Study the drawing (mm; zero at the part's minimum x, y, z) and answer. Coordinates: 2 decimals unless noted, no trailing zeros. Order: outer loops, then holes, each group sorted by start corner. A loop starts at its lowest first (then second) coordinate and runs counter-clockwise, first axis right, second up. Notation, with made-up numbers: M 62.5,73.5 L 67.5,73.5 A14 ccw 67.5,81.5 Z; hole C 86.5,5.25 d10. An arc over 180 degrees is marked long. One line per item, written item: value. Start each with the question number.
Q1. Straight lines are drawn through the part: line 1 along Z through (x, y) = (7, 4.5); line 2 along Z through (x, y) = (1, 4); line 3 along X through (y, z) = (4, 17). For each, find the intervals that lie inside material, in ascending order. Write a range as [from, to].
Q2. The part is cut by section C-C on z = 11.5. Give the vertices of the cut face in (x, y).
Q3. This flat-tipped pin is pushed along its axis until it touches: pin 1 Ø3 at (x, y) = (7, 3) entering from -Z. Where does it stop, or does it pass through?
Q4. The part is cut by section B-B on x = 0.5. Give the number of separate pieces and of enclosed holes in the cut face, then the cut area to 3 significant figures.
Q5. The part is cut by section A-A on y = 2.5. Give the vertices of the cut face in (x, z).
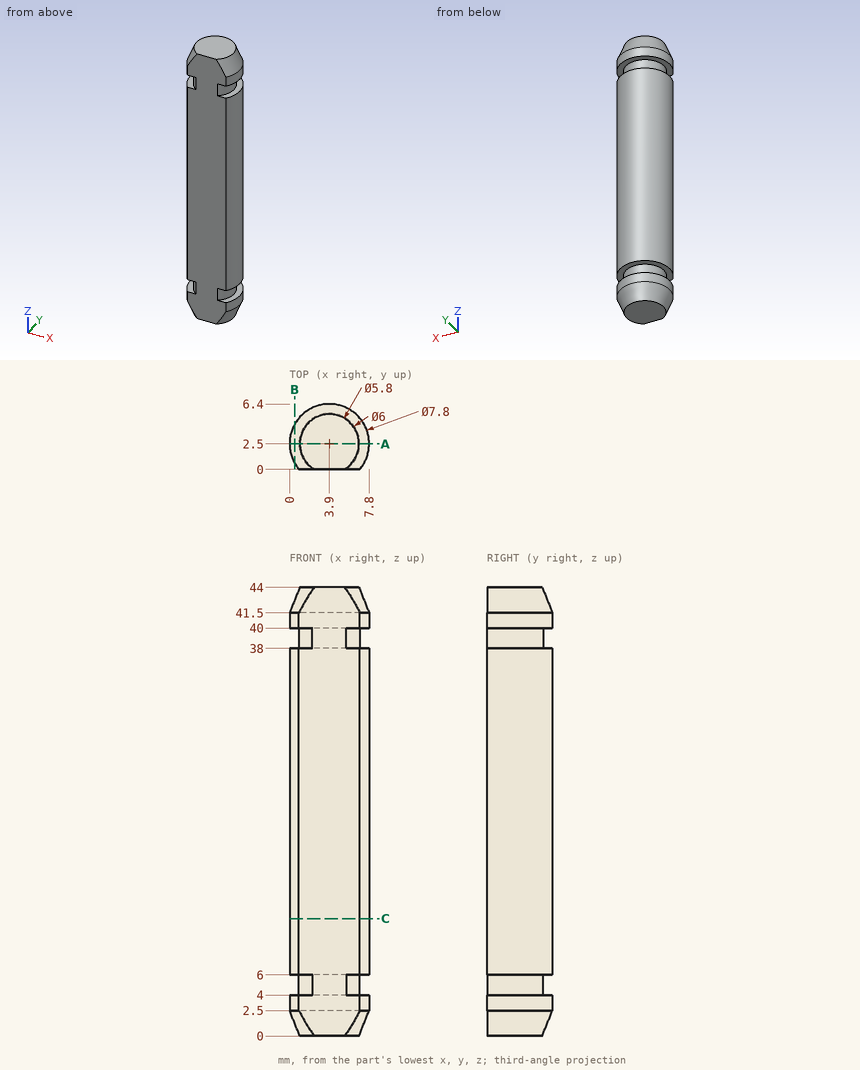
Output:
1. line 1: z = [1.97, 4], [6, 38], [40, 42.03]
1. line 2: z = [0.91, 4], [6, 38], [40, 43.09]
1. line 3: x = [0.3, 7.5]
2. outline: M 0.91,0 L 6.89,0 A3.9 ccw long Z
3. pin 1: stops at z = 0
4. separate pieces: 3
4. enclosed holes: 0
4. area: 140 mm^2
5. outline: M 0,2.5 L 1,0 L 6.8,0 L 7.8,2.5 L 7.8,4 L 6.9,4 L 6.9,6 L 7.8,6 L 7.8,38 L 6.9,38 L 6.9,40 L 7.8,40 L 7.8,41.5 L 6.8,44 L 1,44 L 0,41.5 L 0,40 L 0.9,40 L 0.9,38 L 0,38 L 0,6 L 0.9,6 L 0.9,4 L 0,4 Z
